```python
from build123d import *

# Parameters (mm, degrees)
F0_W      = 50.8
F0_H      = 21.43125
F1_DEPTH  = 1.5875
F2_R      = 1.5875
F3_DEPTH  = 3.175
F5_DEPTH  = 2.38125
F6_W      = 1.5875
F6_H      = 2.38125
F6_W_2    = 5.55625
F6_H_2    = 3.96875
F6_W_3    = 2.38125
F6_H_3    = 3.175
F6_W_4    = 6.35
F6_H_4    = 4.7625
F7_DEPTH  = 1.5875
F8_SIZE   = 0.254
F9_W      = 5.55625
F9_H      = 7.14375
F10_DEPTH = 2.38125
F11_SIZE  = 0.762
F12_SIZE  = 0.254
F13_R     = 5.953125
F14_DEPTH = 9.525
F15_R     = 1.190625
F16_DEPTH = 3.175
F17_W     = 14.2875
F17_H     = 7.14375
F18_DEPTH = 8.73125
F20_DEPTH = 15.24
F22_DEPTH = 11.90625
F23_W     = 3.175
F23_H     = 5.55625
F24_DEPTH = 3.175
F25_W     = 1.5875
F25_H     = 3.175
F26_DEPTH = 1.5875
F27_R     = 0.254
F28_R     = 0.508
F29_W     = 7.9375
F29_H     = 3.175
F30_DEPTH = 3.96875
F31_SIZE  = 0.762


# Not quite as in the source:
# - a length typed as a fraction of an inch, garbled in the dataset ("3 / 203.2 mm" for 3/8 in), is restored


with BuildPart() as f1:
    # F0 (on Top) → F1 (new body)
    with BuildSketch(Plane.XY):
        with Locations((2.7589667588, 1.3157454271)):
            Rectangle(F0_W, F0_H)
    extrude(amount=F1_DEPTH)

    # F2 (on face) → F3 (cut)
    with BuildSketch(Plane.XY.offset(1.5875)):
        with Locations((25.7777167588, -7.0186295729)):
            Circle(F2_R)
        with Locations((25.7777167588, 9.6501204271)):
            Circle(F2_R)
        with Locations((-20.2597832412, 9.6501204271)):
            Circle(F2_R)
        with Locations((-20.2597832412, -7.0186295729)):
            Circle(F2_R)
    extrude(amount=-F3_DEPTH, mode=Mode.SUBTRACT)

    # F4 (on face) → F5 (join)
    with BuildSketch(Plane(origin=(0, 0, 0), x_dir=(1, 0, 0), z_dir=(0, 0, -1))):
        with BuildLine():
            ThreePointArc((-5.1785332412, 6.2248795729), (-5.9722832412, 5.4311295706), (-5.1785332365, 4.6373795729))
            ThreePointArc((-5.1785332365, 4.6373795729), (-4.6172672319, 4.869863567), (-4.3847832412, 5.4311295729))
            ThreePointArc((-4.3847832412, 5.4311295729), (-4.6172672336, 5.9923955805), (-5.1785332412, 6.2248795729))
        make_face()
        with BuildLine():
            ThreePointArc((-2.0035332412, 6.2248795729), (-2.7972832412, 5.4311295729), (-2.0035332412, 4.6373795729))
            ThreePointArc((-2.0035332412, 4.6373795729), (-1.4422672336, 4.8698635653), (-1.2097832412, 5.4311295729))
            ThreePointArc((-1.2097832412, 5.4311295729), (-1.4422672336, 5.9923955805), (-2.0035332412, 6.2248795729))
        make_face()
        with BuildLine():
            ThreePointArc((1.1714667642, 6.2248795729), (0.3777167588, 5.4311295756), (1.1714667588, 4.6373795729))
            ThreePointArc((1.1714667588, 4.6373795729), (1.7327327664, 4.8698635653), (1.9652167588, 5.4311295729))
            ThreePointArc((1.9652167588, 5.4311295729), (1.7327327683, 5.9923955786), (1.1714667642, 6.2248795729))
        make_face()
        with BuildLine():
            ThreePointArc((-7.5597832412, -7.2688704271), (-7.7922672352, -6.7076044179), (-8.3535332458, -6.4751204271))
            ThreePointArc((-8.3535332458, -6.4751204271), (-9.1472832412, -7.2688704294), (-8.3535332412, -8.0626204271))
            ThreePointArc((-8.3535332412, -8.0626204271), (-7.7922672336, -7.8301364347), (-7.5597832412, -7.2688704271))
        make_face()
        with BuildLine():
            ThreePointArc((-4.3085832412, -7.2688704271), (-4.5410672352, -6.7076044179), (-5.1023332458, -6.4751204271))
            ThreePointArc((-5.1023332458, -6.4751204271), (-5.8960832412, -7.2688704294), (-5.1023332412, -8.0626204271))
            ThreePointArc((-5.1023332412, -8.0626204271), (-4.5410672336, -7.8301364347), (-4.3085832412, -7.2688704271))
        make_face()
        with BuildLine():
            ThreePointArc((-1.0573832412, -7.2688704271), (-1.2898672338, -6.7076044193), (-1.8511332418, -6.4751204271))
            ThreePointArc((-1.8511332418, -6.4751204271), (-2.6448832412, -7.2688704205), (-1.8511332549, -8.0626204271))
            ThreePointArc((-1.8511332549, -8.0626204271), (-1.2898672385, -7.8301364395), (-1.0573832412, -7.2688704271))
        make_face()
        with BuildLine():
            ThreePointArc((2.1938167588, -7.2688704271), (1.9613327658, -6.7076044189), (1.4000667571, -6.4751204271))
            ThreePointArc((1.4000667571, -6.4751204271), (0.6063167588, -7.2688704213), (1.4000667456, -8.0626204271))
            ThreePointArc((1.4000667456, -8.0626204271), (1.9613327617, -7.8301364393), (2.1938167588, -7.2688704271))
        make_face()
        with BuildLine():
            ThreePointArc((-8.3535332412, 6.2248795729), (-9.1472832412, 5.4311295729), (-8.3535332412, 4.6373795729))
            ThreePointArc((-8.3535332412, 4.6373795729), (-7.7922672336, 4.8698635653), (-7.5597832412, 5.4311295729))
            ThreePointArc((-7.5597832412, 5.4311295729), (-7.7922672336, 5.9923955805), (-8.3535332412, 6.2248795729))
        make_face()
    extrude(amount=F5_DEPTH)

    # F6 (on face) → F7 (join)
    with BuildSketch(Plane(origin=(0, 0, 0), x_dir=(1, 0, 0), z_dir=(0, 0, -1))):
        with Locations((-15.4972832412, 7.4155045729)):
            Rectangle(F6_W, F6_H)
        with Locations((-15.4972832412, 4.2405045729)):
            Rectangle(F6_W, F6_H)
        with Locations((-13.9097832412, -8.4594954271)):
            Rectangle(F6_W, F6_H)
        with Locations((-6.3691582412, 1.0655045729)):
            Rectangle(F6_W_2, F6_H_2)
        with Locations((0.7745917588, -0.1251204271)):
            Rectangle(F6_W_3, F6_H_3)
        with Locations((18.6339667588, 1.4623795729)):
            Rectangle(F6_W_4, F6_H_4)
        with Locations((18.2370917588, -4.8876204271)):
            Rectangle(F6_W_3, F6_H_4)
    extrude(amount=F7_DEPTH)

    # F8
    f8_edges = [f1.edges().sort_by_distance(p)[0] for p in [
        (-13.909783, 7.26887, -1.5875),
        (-14.703533, 8.459495, -1.5875),
        (-13.909783, 9.65012, -1.5875),
        (-13.116033, 8.459495, -1.5875),
        (-15.497283, -5.43113, -1.5875),
        (-16.291033, -4.240505, -1.5875),
        (-15.497283, -3.04988, -1.5875),
        (-14.703533, -4.240505, -1.5875),
        (-15.497283, -8.60613, -1.5875),
        (-16.291033, -7.415505, -1.5875),
        (-15.497283, -6.22488, -1.5875),
        (-14.703533, -7.415505, -1.5875),
        (-3.591033, -1.065505, -1.5875),
        (-6.369158, -3.04988, -1.5875),
        (-9.147283, -1.065505, -1.5875),
        (-6.369158, 0.91887, -1.5875),
        (0.774592, 1.71262, -1.5875),
        (1.965217, 0.12512, -1.5875),
        (0.774592, -1.46238, -1.5875),
        (-0.416033, 0.12512, -1.5875),
        (18.633967, 0.91887, -1.5875),
        (21.808967, -1.46238, -1.5875),
        (18.633967, -3.84363, -1.5875),
        (15.458967, -1.46238, -1.5875),
        (18.237092, 2.50637, -1.5875),
        (17.046467, 4.88762, -1.5875),
        (18.237092, 7.26887, -1.5875),
        (19.427717, 4.88762, -1.5875),
    ]]
    chamfer(f8_edges, length=F8_SIZE)

    # F9 (on face) → F10 (join)
    with BuildSketch(Plane(origin=(0, 0, 0), x_dir=(1, 0, 0), z_dir=(0, 0, -1))):
        with Locations((7.9183417588, -2.1094954271)):
            Rectangle(F9_W, F9_H)
    extrude(amount=F10_DEPTH)

    # F11
    f11_edges = [f1.edges().sort_by_distance(p)[0] for p in [
        (10.696467, 2.109495, -2.38125),
        (5.140217, 2.109495, -2.38125),
    ]]
    chamfer(f11_edges, length=F11_SIZE)

    # F12
    f12_edges = [f1.edges().sort_by_distance(p)[0] for p in [
        (7.918342, -1.46238, -2.38125),
        (7.918342, 5.68137, -2.38125),
    ]]
    chamfer(f12_edges, length=F12_SIZE)

    # F13 (on face) → F14 (join)
    with BuildSketch(Plane.XY.offset(1.5875)):
        with Locations((-16.6879082412, 1.3157454271)):
            Circle(F13_R)
    extrude(amount=F14_DEPTH)

    # F15 (on face) → F16 (cut)
    with BuildSketch(Plane.XY.offset(11.1125)):
        with Locations((-16.6879082412, 1.3157454271)):
            Circle(F15_R)
    extrude(amount=-F16_DEPTH, mode=Mode.SUBTRACT)

    # F17 (on face) → F18 (join)
    with BuildSketch(Plane.XY.offset(1.5875)):
        with Locations((-3.5910332412, 8.4594954271)):
            Rectangle(F17_W, F17_H)
        with Locations((-3.5910332412, -5.8280045729)):
            Rectangle(F17_W, F17_H)
    extrude(amount=F18_DEPTH)

    # F19 (on face) → F20 (cut)
    with BuildSketch(Plane.YZ.offset(3.5527167588)):
        Polygon((-12.6245096326, 12.3970924459), (-9.3998795729, 7.14375), (-7.8123795729, 10.31875), (-6.8544447422, 13.4305364035), align=None)
        Polygon((11.735675374, 13.160722746), (10.4438704271, 10.31875), (12.0313704271, 7.14375), (15.6484242786, 9.6412404954), (16.4722963069, 13.6774447247), align=None)
    extrude(amount=-F20_DEPTH, mode=Mode.SUBTRACT)

    # F21 (on face) → F22 (join)
    with BuildSketch(Plane.YZ.offset(3.5527167588)):
        with BuildLine():
            ThreePointArc((2.0925854259, 1.6797255876), (3.9220601171, 2.8522266244), (4.6336204271, 4.905375))
            ThreePointArc((4.6336204271, 4.905375), (-0.7374029485, 7.51168969), (0.5389054283, 1.6797255876))
            Line((0.5389054283, 1.6797255876), (2.0925854259, 1.6797255876))
        make_face()
        with BuildLine():
            Line((2.0925854259, 1.6797255876), (0.5389054283, 1.6797255876))
            ThreePointArc((0.5389054283, 1.6797255876), (1.3157454271, 1.5875), (2.0925854259, 1.6797255876))
        make_face()
        with BuildLine():
            ThreePointArc((2.0925854259, 1.6797255876), (1.3157454271, 1.5875), (0.5389054283, 1.6797255876))
            Line((0.5389054283, 1.6797255876), (0.5389054283, 1.5345554566))
            Line((0.5389054283, 1.5345554566), (2.0925854259, 1.5345554566))
            Line((2.0925854259, 1.5345554566), (2.0925854259, 1.6797255876))
        make_face()
    extrude(amount=-F22_DEPTH)

    # F23 (on face) → F24 (join)
    with BuildSketch(Plane.XY.offset(1.5875)):
        with Locations((24.9839667588, 0.5219954271)):
            Rectangle(F23_W, F23_H)
    extrude(amount=F24_DEPTH)

    # F25 (on face) → F26 (join)
    with BuildSketch(Plane.XY.offset(4.7625)):
        with Locations((24.9839667588, 0.5219954271)):
            Rectangle(F25_W, F25_H)
    extrude(amount=F26_DEPTH)

    # F27
    f27_edges = [f1.edges().sort_by_distance(p)[0] for p in [
        (25.777717, -1.065505, 5.55625),
        (24.190217, -1.065505, 5.55625),
        (24.190217, 2.109495, 5.55625),
        (25.777717, 2.109495, 5.55625),
    ]]
    fillet(f27_edges, radius=F27_R)

    # F28
    f28_edges = [f1.edges().sort_by_distance(p)[0] for p in [
        (26.571467, 3.30012, 3.175),
        (23.396467, 3.30012, 3.175),
        (26.571467, -2.25613, 3.175),
        (23.396467, -2.25613, 3.175),
    ]]
    fillet(f28_edges, radius=F28_R)

    # F29 (on face) → F30 (join)
    with BuildSketch(Plane.XY.offset(1.5875)):
        with Locations((9.9027167588, -7.8123795729)):
            Rectangle(F29_W, F29_H)
    extrude(amount=F30_DEPTH)

    # F31
    f31_edges = [f1.edges().sort_by_distance(p)[0] for p in [
        (9.902717, -9.39988, 5.55625),
    ]]
    chamfer(f31_edges, length=F31_SIZE)


solid = f1.part
```
Check sheet for the modelled part. Datum: model origin and axes. Units: mm. A direction names the side the tool comes from. Round coordinates to 2 decimals unless told otherwise and drop trailing zeros. Order: outer loops, then holes, each group sorted by start corner. A loop starts at its lowest first (then second) coordinate and runs counter-clockwise, first axis right, second up. Notation, with made-up numbers: (51, 53) -> (96, 53) arc R29 ccw to (96, 85) -> close; hole circle Ø9 at (-9.75, -27). An arc over 180 degrees is marked (long way). Use CSV: the item, a comma, the result in double quotes.
(1) Depth check by flat-ended pin: pin 1 (1.1 mm diameter, centred on x = 18.5, z = -1, fed in from +Y); pin 2 (10.5 mm diameter, centred on x = 5, y = 2.5, fed in from +Z); pin 3 (1.5 mm diameter, centred on x = 6, y = 9.5, fed in from -Z). Enter the tip coordinate at first touch or a pass-through.
Worked out:
pin 1,"y = 7.27"
pin 2,"z = 10.32"
pin 3,"z = 0"
(2) Draft check along Y on faces 4 (the face through (-15.55, 1.67, 9.55)), 5 (the face through (-3.591, -1, -1)), 6 (the face through (-8.354, 1, 5)), 7 (the face through (-14, 9.65, -1)). Enter one of: pulls with the +Y half, pulls with the -Y half, needs draft (parallel to the pull), parting line crosses it, or undercut.
Worked out:
face 4,"undercut"
face 5,"needs draft"
face 6,"undercut"
face 7,"pulls with the +Y half"
(3) Material ranges on line 1 along Y through (x, z) = (18.5, -1); line 2 along X through (y, z) = (-5.5, -0.75); line 3 along X through (y, z) = (2.5, 3.5), recorded low to high. Write a range as from..to.
Worked out:
line 1,"-3.84..0.92, 2.51..7.27"
line 2,"-9.14..-7.56, -5.97..-4.39, -2.79..-1.21, 0.38..1.96"
line 3,"-22.52..-10.85, -8.35..3.55, 23.4..26.57"
(4) Tool access check on faces 1 (the face through (26, 1, 4.762)), 2 (the face through (26.571, 0, 3)), 3 (the face through (5.934, -8, 4)). Record the directions out of +Z, -Z, +X, -X, +Y, -Y that give a thin tool (end or side, any length) a straight path to the whole face; none if there is none.
Worked out:
face 1,"+Z"
face 2,"+Z, +X, +Y, -Y"
face 3,"+Z, +Y, -Y"
(5) Cross-section at C-C (z = 9.25). Record the boundary of the cut face in (x, y).
Worked out:
outline,"circle Ø11.91 at (-16.69, 1.32); (-10.73, -8.35) -> (3.55, -8.35) -> (3.55, -2.26) -> (-10.73, -2.26) -> close; (-10.73, 4.89) -> (3.55, 4.89) -> (3.55, 10.98) -> (-10.73, 10.98) -> close; hole circle Ø2.38 at (-16.69, 1.32)"
(6) Cross-section at A-A (z = 3.75). Record the boundary of the cut face in (x, y), and give its area (3 significant figures).
Worked out:
outline,"circle Ø11.91 at (-16.69, 1.32); (-10.73, -9.4) -> (3.55, -9.4) -> (3.55, -2.26) -> (-10.73, -2.26) -> close; (-10.73, 4.89) -> (3.55, 4.89) -> (3.55, 12.03) -> (-10.73, 12.03) -> close; (-8.35, -1.79) -> (3.55, -1.79) -> (3.55, 4.43) -> (-8.35, 4.43) -> close; (5.93, -9.4) -> (13.87, -9.4) -> (13.87, -6.22) -> (5.93, -6.22) -> close; (23.4, -1.75) arc R0.51 ccw to (23.9, -2.26) -> (26.06, -2.26) arc R0.51 ccw to (26.57, -1.75) -> (26.57, 2.79) arc R0.51 ccw to (26.06, 3.3) -> (23.9, 3.3) arc R0.51 ccw to (23.4, 2.79) -> close"
area,"432 mm²"
(7) Cross-section at D-D (x = 6.5). Record the boundary of the cut face in (y, z).
Worked out:
outline,"(-9.4, 0) -> (-1.46, 0) -> (-1.46, -2.13) -> (-1.21, -2.38) -> (5.43, -2.38) -> (5.68, -2.13) -> (5.68, 0) -> (12.03, 0) -> (12.03, 1.59) -> (-6.22, 1.59) -> (-6.22, 5.56) -> (-8.64, 5.56) -> (-9.4, 4.79) -> close"
(8) Cross-section at B-B (y = 4). Record the boundary of the cut face in (x, z), and give its area (3 significant figures).
Worked out:
outline,"(-22.64, 0) -> (5.14, 0) -> (5.14, -1.62) -> (5.9, -2.38) -> (9.93, -2.38) -> (10.7, -1.62) -> (10.7, 0) -> (17.05, 0) -> (17.05, -1.33) -> (17.3, -1.59) -> (19.17, -1.59) -> (19.43, -1.33) -> (19.43, 0) -> (28.16, 0) -> (28.16, 1.59) -> (-11.37, 1.59) -> (-11.37, 11.11) -> (-22, 11.11) -> (-22, 1.59) -> (-22.64, 1.59) -> close; (-8.35, 2.96) -> (3.55, 2.96) -> (3.55, 6.86) -> (-8.35, 6.86) -> close"
area,"245 mm²"
